Could you check a few things on this model? Use its own coordinates, in mm. Coordinates: 2 decimals unless noted, no trailing zeros. Loops run counter-clockwise (first coordinate to the right, second up) from the corner with the lowest first, then second, coordinate; pieces in that order, holes last. Notation, with made-up numbers: (48.25, 57) - (97.25, 57) arc R32 ccw to (97.25, 84) - close; hole circle Ø9 at (-24, 8). An arc over 180 degrees is marked (long way). One line per item, written item: value. Start each with the question number.
(1) If I drill on line 1 along Z through (x, y) = (2, -0.25); line 2 along Z through (x, y) = (0, -2); line 3 along Y through (x, z) = (0.75, -25.5), over which ranges is the centre line in solid material (lowest first)? Write a range as from..to.
(2) If we section it at D-D on x = -2.25: Write out the boundary of the cut face in (y, z).
(3) I'm going to push flat-ended pins straight in: P1, Ø3, axis at x = 0.5, z = -16, coming from the +Y side (3 decimals); P2, Ø2, axis at x = 3, y = -2.5, coming from the +Z side; P3, Ø1.1, axis at x = -1.5, y = 0, coming from the -Z side. Where does each tip first touch, or does it pass through?
(4) If we section it at B-B on x = 0: Write out the boundary of the cut face in (y, z) (3 decimals).
(5) If we mould it in two halves opening along Y, with no side actions, what happens to faces 1 (the face through (1, 2, -25.4)), 2 (the face through (0.25, -1.89, -12.88)), 3 (the face through (0, 0, -28.702))? For each: pulls with the +Y half, pulls with the -Y half, needs draft (parallel to the pull), parting line crosses it, or undercut.
(6) If we section it at A-A on y = 0: Write out the boundary of the cut face in (x, z) (3 decimals), then the cut area to 3 significant figures.
(7) If we section it at C-C on z = -8.75: Write out the boundary of the cut face in (x, y) (3 decimals).
```python
from build123d import *

# Parameters (mm, degrees)
CUT_EXTRUDE1_DEPTH = 127


with BuildPart() as part:
    # Sketch2 → Revolve1 (revolve)
    with BuildSketch(Plane(origin=(0, 0, 0), x_dir=(1, 0, 0), z_dir=(0, 1, 0)), mode=Mode.PRIVATE) as revolve1_sk:
        Polygon((0, 0), (1.905, 0), (1.905, 25.4), (4.445, 25.4), (4.445, 29.21), (0, 29.21), align=None)
    revolve(revolve1_sk.sketch.rotate(Axis((0, 0, -29.21), (0, 0, 1)), 180), axis=Axis((0, 0, -29.21), (0, 0, 1)))

    # Sketch3 → Cut-Extrude1 (cut, symmetric)
    with BuildSketch(Plane(origin=(0, 0, 0), x_dir=(0, 0, -1), z_dir=(1, 0, 0))):
        Polygon((29.21, 0.657737685), (29.21, 0), (29.21, -0.762), (28.702, -0.762), (28.702, 0.657737685), align=None)
    extrude(amount=CUT_EXTRUDE1_DEPTH, both=True, mode=Mode.SUBTRACT)


solid = part.part
```
Values:
1. line 1: z = -28.7..-25.4
1. line 2: z = -29.21..-25.4
1. line 3: y = -4.38..4.38
2. outline: (-3.83, -29.21) - (-0.76, -29.21) - (-0.76, -28.7) - (0.66, -28.7) - (0.66, -29.21) - (3.83, -29.21) - (3.83, -25.4) - (-3.83, -25.4) - close
3. P1: stops at y = 1.905
3. P2: stops at z = -25.4
3. P3: stops at z = -28.7
4. outline: (-4.445, -29.21) - (-0.762, -29.21) - (-0.762, -28.702) - (0.658, -28.702) - (0.658, -29.21) - (4.445, -29.21) - (4.445, -25.4) - (1.905, -25.4) - (1.905, 0) - (-1.905, 0) - (-1.905, -25.4) - (-4.445, -25.4) - close
5. face 1: needs draft
5. face 2: parting line crosses it
5. face 3: undercut
6. outline: (-4.445, -28.702) - (4.445, -28.702) - (4.445, -25.4) - (1.905, -25.4) - (1.905, 0) - (-1.905, 0) - (-1.905, -25.4) - (-4.445, -25.4) - close
6. area: 126 mm2
7. outline: circle Ø3.81 at (0, 0)
